The figure shows three views and two pictorial views of one solid part (mm, origin at its lowest corner). Answer the questions. Coordinates: 2 decimals unless noted, no trailing zeros. Loops run counter-clockwise (first coordinate to the right, second up) from the corner with the lowest first, then second, coordinate; pieces in that order, holes last. Notation, with made-up numbers: (75, 9.25) -> (91, 9.25) arc R25 cw to (91, 42.25) -> close; hole circle Ø7 at (61.5, -9.5). An arc over 180 degrees is marked (long way). Answer in a Markdown table with one row per item.
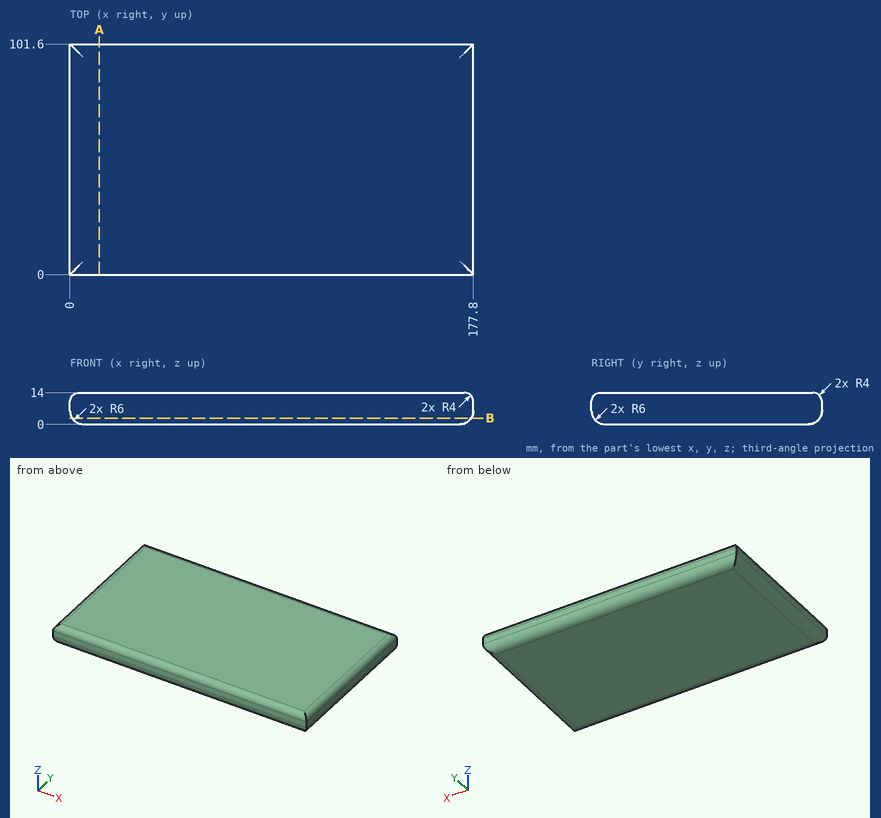
Item 1: A cutting plane is placed at B-B, the plane z = 2.75. Determine the outline of the cut face in (x, y), plus the area to 3 significant figures.
Findings below:
| item | result |
|---|---|
| outline | (0.96, 0.96) -> (176.84, 0.96) -> (176.84, 100.64) -> (0.96, 100.64) -> close |
| area | 17,500 mm2 |
Item 2: Flat-ended cylindrical pins translate along their axes: pin 1 Ø8 at (x, y) = (72, 73) entering from -Z; pin 2 Ø3 at (y, z) = (89, 12.5) entering from -X. Find the tip coordinate at first contact, or state that the pin passes through.
Findings below:
| item | result |
|---|---|
| pin 1 | stops at z = 0 |
| pin 2 | stops at x = 0.13 |
Item 3: Find the intervals of material crossed by probe 1 along X at (y, z) = (24.5, 5.5); probe 2 along Y at (x, z) = (71.5, 5.5); probe 3 along Z at (x, y) = (44, 5.5), in increasing order.
Findings below:
| item | result |
|---|---|
| probe 1 | x = 0.02 to 177.78 |
| probe 2 | y = 0.02 to 101.58 |
| probe 3 | z = 0.02 to 14 |
Item 4: A cutting plane is placed at A-A, the plane x = 13. Determine the outline of the cut face in (y, z), plus the area to 3 significant figures.
Findings below:
| item | result |
|---|---|
| outline | (0, 6) arc R6 ccw to (6, 0) -> (95.6, 0) arc R6 ccw to (101.6, 6) -> (101.6, 10) arc R4 ccw to (97.6, 14) -> (4, 14) arc R4 ccw to (0, 10) -> close |
| area | 1,400 mm2 |
